Input: part model. Units: mm. Frame: model coordinates. A direction names the side the tool comes from. Round coordinates to 2 decimals unless told otherwise and drop trailing zeros. Write each loop counter-clockwise with the first axis right and the second up, starting at its lowest first coordinate (ties: lowest second). Pieces come first, ordered by that corner, then holes. Notation, with made-up numbers: M 39,41.5 L 68,41.5 A15 cw 68,68.5 Z; hole C 44,67.25 d6. An arc over 180 degrees is marked long. Answer as CSV lines item,"result". Start each with the question number.
```python
from build123d import *

# Parameters (mm, degrees)
SKETCH1_R           = 15
BOSS_EXTRUDE1_DEPTH = 20
SKETCH2_R           = 7.5
CUT_EXTRUDE1_DEPTH  = 10
SKETCH3_W           = 25
SKETCH3_H           = 8.533910502
BOSS_EXTRUDE2_DEPTH = 30
SKETCH4_R           = 5
CUT_EXTRUDE2_DEPTH  = 30
SKETCH5_R           = 7.5
BOSS_EXTRUDE3_DEPTH = 15


with BuildPart() as part:
    # Sketch1 → Boss-Extrude1 (new body)
    with BuildSketch(Plane(origin=(0, 0, 0), x_dir=(1, 0, 0), z_dir=(0, 1, 0))):
        Circle(SKETCH1_R)
    extrude(amount=BOSS_EXTRUDE1_DEPTH)

    # Sketch2 → Cut-Extrude1 (cut)
    with BuildSketch(Plane.XZ):
        Circle(SKETCH2_R)
    extrude(amount=-CUT_EXTRUDE1_DEPTH, mode=Mode.SUBTRACT)

    # Sketch3 → Boss-Extrude2 (add)
    with BuildSketch(Plane(origin=(0, 20, 0), x_dir=(1, 0, 0), z_dir=(0, 1, 0))):
        Rectangle(SKETCH3_W, SKETCH3_H)
    extrude(amount=BOSS_EXTRUDE2_DEPTH)

    # Sketch4 → Cut-Extrude2 (cut)
    with BuildSketch(Plane(origin=(0, 0, -4.266955251), x_dir=(-1, 0, 0), z_dir=(0, 0, -1))):
        with Locations((0, 40)):
            Circle(SKETCH4_R)
        with BuildLine():
            Line((12, 112.846805037), (20.699554593, 68.640446889))
            Line((20.699554593, 68.640446889), (12, 40))
            ThreePointArc((12, 40), (0, 52), (-12, 40))
            Line((-12, 40), (-18.346894815, 40))
            Line((-18.346894815, 40), (-15.704364739, 112.846805037))
            Line((-15.704364739, 112.846805037), (12, 112.846805037))
        make_face()
    extrude(amount=-CUT_EXTRUDE2_DEPTH, mode=Mode.SUBTRACT)

    # Sketch5 → Boss-Extrude3 (add)
    with BuildSketch(Plane.XZ.offset(-10)):
        Circle(SKETCH5_R)
    extrude(amount=BOSS_EXTRUDE3_DEPTH)


solid = part.part
```
Item 1: Draft query along X for faces 1 (the face through (-12.253, 40.835, -0.06)), 2 (the face through (10.534, 45.747, -0.06)), 3 (the face through (-0.2, 34.8, -4.267)). Return one class per face: +X half, -X half, draft (parallel to the pull), parting line (faces both ways), or undercut.
Item 2: Cut plane A-A, the plane x = 0. Return loops of the section in (y, z), plus the area to 3 significant figures.
Item 3: Access query for faces 4 (the face through (12.5, 30, 0)), 5 (the face through (-7.493, -2.465, 0.33)), 6 (the face through (-0.2, 34.8, 4.267)), 7 (the face through (-12.5, 31, 0)), 8 (the face through (0, -5, 0)). Directions: +Z, -Z, +X, -X, +Y, -Y. A direction counts if a zero-diameter tool reaches every point of the face in a straight line with its end or side. Return the directions, or none.
Item 4: Line query: line 1 (Y direction, x = 0, z = -1); line 2 (Z direction, x = 9.25, y = 35.5); line 3 (X direction, y = 21.5, z = -1.5). Output: solid intervals per line, ascending. Write a range as [from, to].
Item 5: Cut plane C-C, the plane z = -6.5. Return loops of the section in (x, y), plus the area to 3 significant figures.
Item 6: Pin query (flat end, axial travel): pin 1 Ø11.5 at (x, y) = (0, 40) entering from -Z; pin 2 Ø3 at (x, z) = (9, 8) entering from +Y; pin 3 Ø1.5 at (y, z) = (33.5, -3.5) entering from -X; pin 4 Ø5 at (y, z) = (43, 9) entering from -X. Return the tip coordinate at first contact, or that it passes through.
Item 7: Cut plane D-D, the plane x = 9.5. Return loops of the section in (y, z).
Item 8: Cut plane B-B, the plane z = 0. Return loops of the section in (x, y), plus the area to 3 significant figures.
Results list:
1,face 1,"undercut"
1,face 2,"+X half"
1,face 3,"draft"
2,outline,"M -5,-7.5 L 0,-7.5 L 0,-15 L 20,-15 L 20,-4.27 L 35,-4.27 L 35,4.27 L 20,4.27 L 20,15 L 0,15 L 0,7.5 L -5,7.5 Z; M 45,-4.27 L 50,-4.27 L 50,4.27 L 45,4.27 Z"
2,area,"846 mm²"
3,face 4,"+Z, -Z, +X, +Y"
3,face 5,"-Y"
3,face 6,"+Z, +X, -X, +Y"
3,face 7,"+Z, -Z, -X, +Y"
3,face 8,"+Z, -Z, +X, -X, -Y"
4,line 1,"[-5, 35], [45, 50]"
4,line 2,"[-4.27, 4.27]"
4,line 3,"[-12.5, 12.5]"
5,outline,"M -13.52,0 L -3.74,0 L -3.74,-5 L 3.74,-5 L 3.74,0 L 13.52,0 L 13.52,20 L -13.52,20 Z"
5,area,"578 mm²"
6,pin 1,"z = -4.27"
6,pin 2,"y = 20"
6,pin 3,"x = -12.5"
6,pin 4,"through"
7,outline,"M 0,-11.61 L 20,-11.61 L 20,-4.27 L 47.33,-4.27 L 47.33,4.27 L 20,4.27 L 20,11.61 L 0,11.61 Z"
8,outline,"M -15,0 L -7.5,0 L -7.5,-5 L 7.5,-5 L 7.5,0 L 15,0 L 15,20 L 12.5,20 L 12.5,40 L 12,40 A12 ccw 6.63,50 L -6.63,50 A12 ccw -12,40 L -12.5,41.65 L -12.5,20 L -15,20 Z; hole C 0,40 d10"
8,area,"1,310 mm²"
